Read the model definition and answer for the solid it produces. Units are mm, in the model's axes. Face numbers are marked on the shaded views. A direction names the side the tool comes from. Coordinates: 2 decimals unless noted, no trailing zeros. Loops run counter-clockwise (first coordinate to the right, second up) from the corner with the lowest first, then second, coordinate; pieces in that order, holes last.
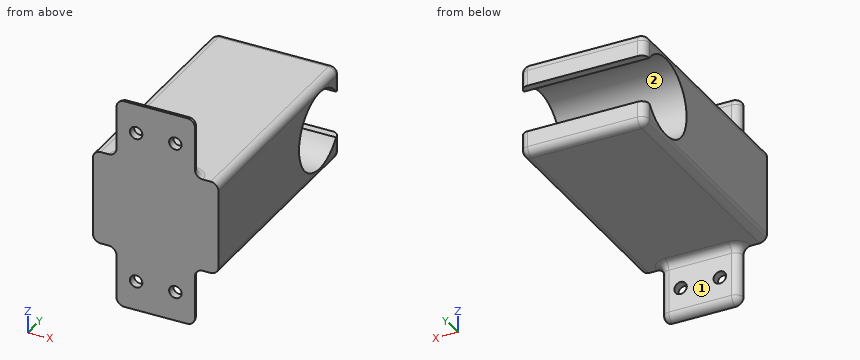
Autodesk Inventor part; units mm, degrees
ref_plane "YZ Plane" through (0, 0, 0) normal (1, 0, 0) x (0, 1, 0)
ref_plane "XZ Plane" through (0, 0, 0) normal (0, 1, 0) x (-1, 0, 0)
ref_plane "XY Plane" through (0, 0, 0) normal (0, 0, 1) x (1, 0, 0)
sketch "Sketch1" plane through (0, 0, 0) normal (0, 1, 0) x (-1, 0, 0)
  line L0 (16, -12) -> (-16, -12)
  line L1 (-16, -12) -> (-16, 12)
  line L2 (-16, 12) -> (16, 12)
  line L3 (16, 12) -> (16, -12)
  line L4 (16, -12) -> (-16, 12) construction
  line L5 (-16, -12) -> (16, 12) construction
  line L6 (-10, 27) -> (10, 27)
  line L7 (10, 27) -> (10, -27)
  line L8 (10, -27) -> (-10, -27)
  line L9 (-10, -27) -> (-10, 27)
  line L10 (-10, 27) -> (10, -27) construction
  line L11 (10, 27) -> (-10, -27) construction
  circle A0 centre (5, 19.5) radius 1.5875
  circle A1 centre (5, -19.5) radius 1.5875
  circle A2 centre (-5, 19.5) radius 1.5875
  circle A3 centre (-5, -19.5) radius 1.5875
  point P0 (0, 0)
  dimension "d0" = 32
  dimension "d1" = 24
  dimension "d2" = 20
  dimension "d3" = 54
  dimension "d4" = 3.175
  dimension "d5" = 7.5
  dimension "d7" = 5
  dimension "d10" = 39
  dimension "d13" = 10
extrude "Extrusion1" add sketch "Sketch1" along normal blind 2
sketch "Sketch2" plane through (0, 2, 0) normal (0, 1, 0) x (1, 0, 0)
  line L0 (16, 12) -> (16, -12)
  line L1 (-16, -12) -> (16, -12)
  line L2 (16, -12) -> (16, 12)
  line L3 (16, 12) -> (-16, 12)
  line L4 (-16, 12) -> (-16, -12)
  line L5 (-16, -12) -> (16, 12) construction
  line L6 (16, -12) -> (-16, 12) construction
  point P0 (0, 0)
extrude "Extrusion2" add sketch "Sketch2" along normal blind 57.15
sketch "Sketch3" plane through (16, 0, 12) normal (1, 0, 0) x (0, 0, -1)
  line L0 (0, 59.15) -> (24, 59.15)
  line L1 (24, 0) -> (0, 0)
  line L2 (24, 0) -> (24, 59.15)
  line L3 (0, 59.15) -> (24, 59.15)
  line L4 (0, 0) -> (0, 59.15)
  circle A0 centre (12, 49.15) radius 10
  point P0 (12, 0)
  dimension "d20" = 20
  dimension "d21" = 10
extrude "Extrusion3" cut sketch "Sketch3" against normal through all contours A0
sketch "Sketch4" plane through (16, 0, 12) normal (1, 0, 0) x (0, 0, -1)
  circle A0 centre (12, 49.15) radius 10
  line L0 (0, 59.15) -> (12, 59.15)
  line L1 (12, 59.15) -> (24, 59.15)
  line L2 (12, 59.15) -> (0, 59.15)
  line L3 (6, 59.15) -> (18, 59.15)
  line L4 (18, 59.15) -> (18, 57.15)
  line L5 (18, 57.15) -> (6, 57.15)
  line L6 (6, 57.15) -> (6, 59.15)
  point P0 (12, 0)
extrude "Extrusion4" cut sketch "Sketch4" against normal through all contours L5 A0 | A0 L1 L4 | L6 L0 A0 picked at (10.6135, 57.5146)
fillet "Fillet1" radius 2 1 edges at (0, 59.15, 12)
fillet "Fillet2" radius 2 1 edges at (0, 59.15, -12)
fillet "Fillet3" radius 2 3 edges at (16, 58.5642, 11.4142) (16, 59.15, 8) (16, 28.575, 12)
fillet "Fillet4" radius 2 3 edges at (16, 58.5642, -11.4142) (16, 59.15, -8) (16, 28.575, -12)
fillet "Fillet5" radius 2 1 edges at (10, 1, 27)
fillet "Fillet6" radius 2 1 edges at (10, 1, -27)
fillet "Fillet7" radius 2 1 edges at (-10, 1, 27)
fillet "Fillet8" radius 2 1 edges at (-10, 1, -27)
fillet "Fillet9" radius 2 3 edges at (-16, 28.575, -12) (-16, 58.5642, -11.4142) (-16, 59.15, -8)
fillet "Fillet10" radius 2 3 edges at (-16, 28.575, 12) (-16, 58.5642, 11.4142) (-16, 59.15, 8)
fillet "Fillet11" radius 2 5 edges at (10, 2, 18.5) (9.4142, 2, 26.4142) (0, 2, 27) (-9.4142, 2, 26.4142) (-10, 2, 18.5)
fillet "Fillet12" radius 2 3 edges at (0, 2, 12) (-9.4144, 1.4144, 12) (9.4144, 1.4144, 12)
fillet "Fillet13" radius 2 5 edges at (0, 2, -27) (-9.4142, 2, -26.4142) (-10, 2, -18.5) (9.4142, 2, -26.4142) (10, 2, -18.5)
fillet "Fillet14" radius 2 3 edges at (0, 2, -12) (9.4144, 1.4144, -12) (-9.4144, 1.4144, -12)
Q1. Which of the six approach directions +Z, -Z, +X, -X, +Y, -Y give full straight-line access (tool end or side, diameter ignored) to the marked faces 1 and 2?
Findings below:
face 1: -Z, +X, -X, +Y
face 2: +X, -X
Q2. A cutting plane is placed at B-B (z = 19.5). Count the separate pieces of the cut face and the enclosed holes in it, then the cut area to 3 significant figures.
Findings below:
separate pieces: 3
enclosed holes: 0
area: 25.6 mm2
Q3. Straight lines are drawn through the part: probe 1 along X at (y, z) = (1, 19); probe 2 along Z at (x, y) = (-5, 1.6); probe 3 along Z at (x, y) = (-1, 49). For each, find the intervals that lie inside material, in ascending order.
Findings below:
probe 1: x = -9.73 to -6.51, -3.49 to 3.49, 6.51 to 9.73
probe 2: z = -26.2 to -21.09, -17.91 to 17.91, 21.09 to 26.2
probe 3: z = -12 to -10, 10 to 12
Q4. A cutting plane is placed at D-D (z = -7.5). Give the vertices of the cut face in (x, y).
Findings below:
outline: (-16, 0) - (16, 0) - (16, 42.54) - (-16, 42.54) - close; (-16, 55.76) - (16, 55.76) - (16, 57.15) arc R2 ccw to (14, 59.15) - (-14, 59.15) arc R2 ccw to (-16, 57.15) - close
Q5. Flat-ended cylindrical pins translate along their axes: pin 1 Ø10 at (x, y) = (-6, 9) entering from +Z; pin 2 Ø4 at (x, z) = (-7.5, 20) entering from -Y; pin 3 Ø4 at (x, z) = (5, -19.5) entering from +Y; pin 4 Ø8.5 at (x, y) = (6, 26) entering from -Z. Find the tip coordinate at first contact, or state that the pin passes through.
Findings below:
pin 1: stops at z = 12
pin 2: stops at y = 0
pin 3: stops at y = 2
pin 4: stops at z = -12
